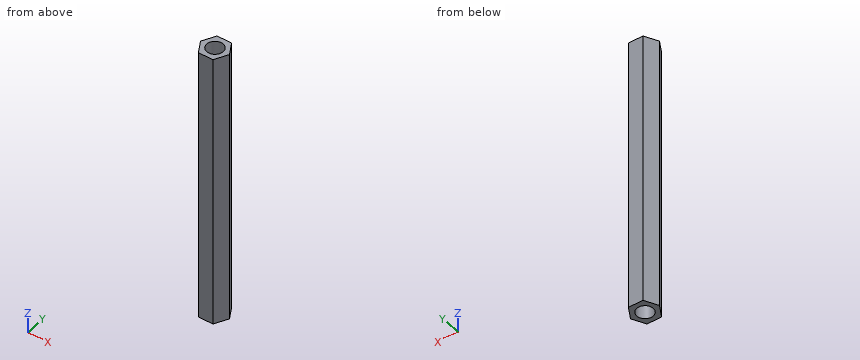
from build123d import *

# Parameters (mm, degrees)
EXTRUDE_1_DEPTH     = 50
SKETCH_2_R          = 1.5
CUT_EXTRUDE_1_DEPTH = 50


with BuildPart() as part:
    # 草图1 → 凸台-拉伸1 (new body)
    with BuildSketch(Plane.XY):
        Polygon((0, 0), (2.675718911, 0), (4.013578367, -2.317240551), (2.796233264, -4.7), (0.120514353, -4.7), (-1.217345103, -2.382759449), align=None)
    extrude(amount=EXTRUDE_1_DEPTH)

    # 草图2 → 切除-拉伸1 (cut)
    with BuildSketch(Plane.XY):
        with Locations((1.398116632, -2.35)):
            Circle(SKETCH_2_R)
    extrude(amount=CUT_EXTRUDE_1_DEPTH, mode=Mode.SUBTRACT)


solid = part.part
Can you work these out from the model? Positions are in its coordinate system, mm. Round coordinates to 2 decimals unless told otherwise and drop trailing zeros. Write each loop counter-clockwise with the first axis right and the second up, starting at its lowest first coordinate (ties: lowest second). Pieces come first, ordered by that corner, then holes. Notation, with made-up numbers: (75, 14) -> (120, 14) arc R12 cw to (120, 30) -> close; hole circle Ø3 at (8, -13). An arc over 180 degrees is marked (long way). One line per question, with ' | ' between items. Start each with the question number.
1) Suppose I cut it at C-C on x = 3.45. Write out the boundary of the cut face in (y, z), then the cut area to 3 significant figures.
2) I need wall thicknesses on line 1 (Y direction, x = 1.3, z = 37.5); line 2 (X direction, y = -2.05, z = 29); line 3 (Y direction, x = 0.85, z = 13.5). Which ranges of each line are inside material? Lowest first, please. Write a range as [from, to].
3) I'm going to push a flat-ended pin straight in: P1, Ø1, axis at y = -1, z = 6.5, coming from the -X side. Where does the tip first touch, or does it pass through?
4) Suppose I cut it at B-B on x = 1.3. Write out the boundary of the cut face in (y, z).
5) Suppose I cut it at A-A on z = 23.5. Write out the boundary of the cut face in (x, y), then the cut area to 3 significant figures.
Return value:
1) outline: (-3.42, 0) -> (-1.34, 0) -> (-1.34, 50) -> (-3.42, 50) -> close | area: 104 mm2
2) line 1: y = [-4.7, -3.85], [-0.85, 0] | line 2: x = [-1.05, -0.07], [2.87, 3.86] | line 3: y = [-4.7, -3.75], [-0.95, 0]
3) P1: stops at x = -0.77
4) outline: (-4.7, 0) -> (-3.85, 0) -> (-3.85, 50) -> (-4.7, 50) -> close; (-0.85, 0) -> (0, 0) -> (0, 50) -> (-0.85, 50) -> close
5) outline: (-1.22, -2.38) -> (0.12, -4.7) -> (2.8, -4.7) -> (4.01, -2.32) -> (2.68, 0) -> (0, 0) -> close; hole circle Ø3 at (1.4, -2.35) | area: 11.5 mm2
